Check sheet for the modelled part. Datum: model origin and axes. Units: mm. Face numbers are marked on the shaded views. A direction names the side the tool comes from. Give positions to 0.01 mm unless a question says otherwise; leave off trailing zeros. Write each loop counter-clockwise with the first axis right and the second up, starting at its lowest first coordinate (ties: lowest second). Pieces come first, ordered by that corner, then holes. Notation, with made-up numbers: M 18,73.5 L 70,73.5 A10 cw 70,79.5 Z; hole C 16.5,39 d4. An arc over 180 degrees is marked long. Write item = value, one per line. Start each with the question number.
1) Scan lines: L1, parallel to Z at x = -20, y = -28; L2, parallel to X at y = -12, z = 17.5; L3, parallel to Y at x = -15, z = 22.5. Record each from-to range of solid material in increasing order.
2) Draft check along Y on the marked faces 3, 4, 5 and 6. Enter one of: pulls with the +Y half, pulls with the -Y half, needs draft (parallel to the pull), parting line crosses it, or undercut.
3) Sectioned sample at A-A, the plane y = 22.5. Record the cut outline in (x, z), then the cut area to 3 significant figures.
4) Sectioned sample at D-D, the plane x = -10. Record the cut outline in (y, z), then the cut area to 3 significant figures.
5) Sectioned sample at B-B, the plane z = 4.5. Record the cut outline in (x, y), then the cut area to 3 significant figures.
6) Set-up check for the marked faces 1 and 2: record each of +Z, -Z, +X, -X, +Y, -Y from which the full face is reachable in a straight line by a thin tool's end or side.
7) Gauge pin test, flat ends, axial feed: pin 1 (13.5 mm diameter, centred on x = -4, y = 7, fed in from +Z); pin 2 (12 mm diameter, centred on x = 17, y = -3, fed in from -Z). Record the tip position at first contact, or that the pin passes through.
8) Sectioned sample at C-C, the plane x = -19. Record the cut outline in (y, z), then the cut area to 3 significant figures.
from build123d import *

# Parameters (mm, degrees)
F0_W     = 50.8
F0_H     = 76.2
F1_DEPTH = 25.4
F2_W     = 25.4
F2_H     = 63.5
F3_DEPTH = 12.7
F4_T     = -2.54


with BuildPart() as f1:
    # F0 (on Top) → F1 (new body)
    with BuildSketch(Plane.XY):
        Rectangle(F0_W, F0_H)
    extrude(amount=F1_DEPTH)

    # F2 (on face) → F3 (cut)
    with BuildSketch(Plane.XY.offset(25.4)):
        Rectangle(F2_W, F2_H)
    extrude(amount=-F3_DEPTH, mode=Mode.SUBTRACT)

    # F4
    f4_openings = [f1.faces().sort_by_distance(p)[0] for p in [
        (-12.7, 0, 19.05),
        (0, 0, 12.7),
        (0, 31.75, 19.05),
        (12.7, 0, 19.05),
        (0, -31.75, 19.05),
    ]]
    offset(amount=F4_T, openings=f4_openings)


solid = f1.part
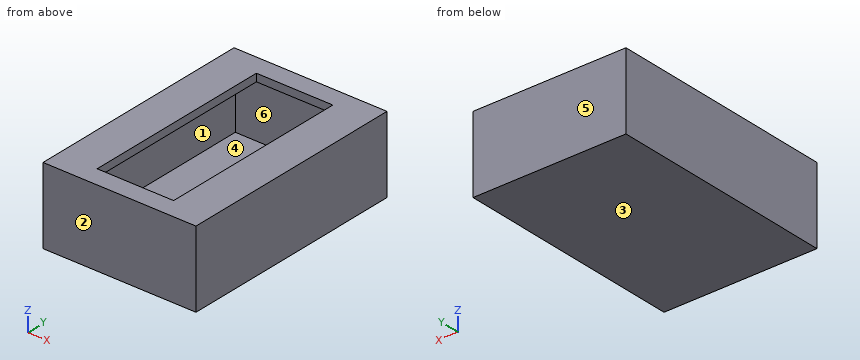
Data:
q1.L1 = 0 to 2.54, 22.86 to 25.4
q1.L2 = -25.4 to -22.86, 22.86 to 25.4
q1.L3 = -38.1 to -35.56, 35.56 to 38.1
q2.face_3 = needs draft
q2.face_4 = undercut
q2.face_5 = pulls with the +Y half
q2.face_6 = undercut
q3.outline = M -25.4,0 L 25.4,0 L 25.4,25.4 L 12.7,25.4 L 12.7,22.86 L 22.86,22.86 L 22.86,2.54 L -22.86,2.54 L -22.86,22.86 L -12.7,22.86 L -12.7,25.4 L -25.4,25.4 Z
q3.area = 297 mm2
q4.outline = M -38.1,0 L 38.1,0 L 38.1,25.4 L 31.75,25.4 L 31.75,22.86 L 35.56,22.86 L 35.56,2.54 L -35.56,2.54 L -35.56,22.86 L -31.75,22.86 L -31.75,25.4 L -38.1,25.4 Z
q4.area = 329 mm2
q5.outline = M -25.4,-38.1 L 25.4,-38.1 L 25.4,38.1 L -25.4,38.1 Z; hole M -22.86,-35.56 L 22.86,-35.56 L 22.86,35.56 L -22.86,35.56 Z
q5.area = 619 mm2
q6.face_1 = none
q6.face_2 = +Z, -Z, +X, -X, -Y
q7.pin_1 = 2.54
q7.pin_2 = 0
q8.outline = M -38.1,0 L 38.1,0 L 38.1,25.4 L -38.1,25.4 Z; hole M -35.56,2.54 L 35.56,2.54 L 35.56,22.86 L -35.56,22.86 Z
q8.area = 490 mm2
